Work out the finished part from the listing and answer in its coordinate system (mm). Face numbers are marked on the shaded views. A direction names the side the tool comes from. Coordinates: 2 decimals unless noted, no trailing zeros. Write each loop counter-clockwise with the first axis right and the second up, starting at its lowest first coordinate (ties: lowest second). Pieces come first, ordered by that corner, then holes. Notation, with made-up numbers: (-34, -16.5) - (18, -16.5) arc R28 ccw to (18, 4.5) - close; hole circle Ø9 at (-4.5, 16). An arc over 180 degrees is marked (long way). Use a Markdown table: item, result. Add a question column.
(1) The part is cut by section D-D, the plane x = 28. Give the vertices of the cut face in (y, z), then the cut area to 4 significant figures.
(2) The part is cut by section A-A, the plane x = 22. Give the vertices of the cut face in (y, z).
(3) For a pull along X with two mould halves and no side action, classify the marked faces 1, 2, 3 and 4 as released by +X, released by -X, zero draft, split by the parting line, or undercut.
(4) Find the intervals of material crossed by line 1 (Y direction, x = 13, z = 1.2); line 2 (Z direction, x = 17, y = 21); line 3 (X direction, y = 22.25, z = 3.9), in increasing order. Write a range as from..to.
(5) The part is cut by section C-C, the plane z = 4.35. Give the vertices of the cut face in (x, y), then the cut area to 3 significant figures.
(6) A tool of negligible diameter and unlimited length cuts with its end or side. For the marked faces 5 and 6, from which of +Z, -Z, +X, -X, +Y, -Y can it reach the whole face along a straight path? Write none if from no direction.
(7) Given pin 1 Ø1 at (x, y) = (27, 21.5) entering from -Z; pin 2 Ø0.7 at (y, z) = (18, 4) entering from +X; pin 3 Ø1.5 at (y, z) = (16.5, 1) entering from +X; pin 4 Ø1.9 at (y, z) = (18, 4) entering from -X, each flat-ended and moving along its own axis, determine where each tip first touches the part or whether it passes through.
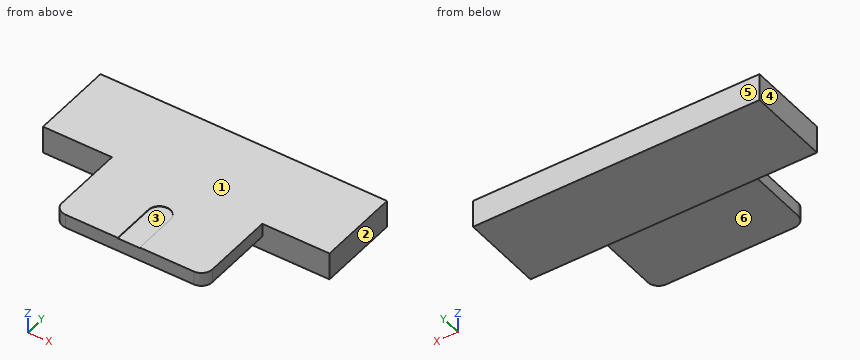
from build123d import *

# Parameters (mm, degrees)
BOX033_W          = 27.28
BOX033_H          = 15
BOX033_DEPTH      = 2.4
BOX031_W          = 10
BOX031_H          = 15
BOX031_DEPTH      = 5
BOX032_W          = 10
BOX032_H          = 15
BOX032_DEPTH      = 5
BOX030_W          = 4
BOX030_H          = 16
BOX030_DEPTH      = 10
CYLINDER023_R     = 2
CYLINDER023_DEPTH = 10
BOX029_W          = 8.2
BOX029_H          = 15
BOX029_DEPTH      = 10
BOX028_W          = 8.52
BOX028_H          = 15
BOX028_DEPTH      = 10
BOX027_W          = 44
BOX027_H          = 15
BOX027_DEPTH      = 2.6
BOX026_W          = 44
BOX026_H          = 30
BOX026_DEPTH      = 5
FILLET006_R       = 2


with BuildPart() as cube033:
    # Box033 → Box033 (new body)
    with BuildSketch(Plane(origin=(8.5, 21, 2.5), x_dir=(1, 0, 0), z_dir=(0, 0, 1))):
        with Locations((13.64, 7.5)):
            Rectangle(BOX033_W, BOX033_H)
    extrude(amount=BOX033_DEPTH)


with BuildPart() as cube031:
    # Box031 → Box031 (new body)
    with BuildSketch(Plane(origin=(-4, 36, 0), x_dir=(1, 0, 0), z_dir=(0, 0, 1))):
        with Locations((5, 7.5)):
            Rectangle(BOX031_W, BOX031_H)
    extrude(amount=BOX031_DEPTH)


with BuildPart() as cube032:
    # Box032 → Box032 (new body)
    with BuildSketch(Plane(origin=(38, 36, 0), x_dir=(1, 0, 0), z_dir=(0, 0, 1))):
        with Locations((5, 7.5)):
            Rectangle(BOX032_W, BOX032_H)
    extrude(amount=BOX032_DEPTH)


with BuildPart() as cube030:
    # Box030 → Box030 (new body)
    with BuildSketch(Plane(origin=(20, -8, 0), x_dir=(1, 0, 0), z_dir=(0, 0, 1))):
        with Locations((2, 8)):
            Rectangle(BOX030_W, BOX030_H)
    extrude(amount=BOX030_DEPTH)


with BuildPart() as fusion024:
    # Cylinder023 → Cylinder023 (new body)
    with BuildSketch(Plane(origin=(22, 8, 0), x_dir=(1, 0, 0), z_dir=(0, 0, 1))):
        Circle(CYLINDER023_R)
    extrude(amount=CYLINDER023_DEPTH)

    # Fusion024: union Cube030
    add(cube030.part)


with BuildPart() as cube029:
    # Box029 → Box029 (new body)
    with BuildSketch(Plane(origin=(35.8, 0, 0), x_dir=(1, 0, 0), z_dir=(0, 0, 1))):
        with Locations((4.1, 7.5)):
            Rectangle(BOX029_W, BOX029_H)
    extrude(amount=BOX029_DEPTH)


with BuildPart() as cube028:
    # Box028 → Box028 (new body)
    with BuildSketch(Plane.XY):
        with Locations((4.26, 7.5)):
            Rectangle(BOX028_W, BOX028_H)
    extrude(amount=BOX028_DEPTH)


with BuildPart() as cube027:
    # Box027 → Box027 (new body)
    with BuildSketch(Plane.XY):
        with Locations((22, 7.5)):
            Rectangle(BOX027_W, BOX027_H)
    extrude(amount=BOX027_DEPTH)


with BuildPart() as exterior_parte2_v2_base:
    # Box026 → Box026 (new body)
    with BuildSketch(Plane.XY):
        with Locations((22, 15)):
            Rectangle(BOX026_W, BOX026_H)
    extrude(amount=BOX026_DEPTH)

    # Cut007002012: cut Cube027
    add(cube027.part, mode=Mode.SUBTRACT)

    # Cut007002013: cut Cube028
    add(cube028.part, mode=Mode.SUBTRACT)

    # Cut007002014: cut Cube029
    add(cube029.part, mode=Mode.SUBTRACT)

    # Cut007002015: cut Fusion024
    add(fusion024.part, mode=Mode.SUBTRACT)


with BuildPart() as exterior_parte2_v2_base_1:
    # Cut007002015 placement: moved
    add(exterior_parte2_v2_base.part.moved(Location((0, 21, 0))))

    # Fusion025: union Cube031, Cube032
    add(cube031.part)
    add(cube032.part)

    # Fusion026: union Cube033
    add(cube033.part)

    # Fillet006
    fillet006_edges = [exterior_parte2_v2_base_1.edges().sort_by_distance(p)[0] for p in [
        (8.5, 21, 3.7),
        (35.8, 21, 3.8),
    ]]
    fillet(fillet006_edges, radius=FILLET006_R)


with BuildPart() as exterior_parte2_v2_base_2:
    # Fillet006 placement: moved
    add(exterior_parte2_v2_base_1.part.moved(Location((0, -12, 0.05))))


solid = exterior_parte2_v2_base_2.part
Model answer:
| question | item | result |
|---|---|---|
| 1 | outline | (9, 2.55) - (24, 2.55) - (24, 0.05) - (39, 0.05) - (39, 5.05) - (9, 5.05) - close |
| 1 | area | 112.5 mm^2 |
| 2 | outline | (9, 2.55) - (24, 2.55) - (24, 0.05) - (39, 0.05) - (39, 5.05) - (19, 5.05) - (19, 4.95) - (9, 4.95) - close |
| 3 | face 1 | zero draft |
| 3 | face 2 | released by +X |
| 3 | face 3 | undercut |
| 3 | face 4 | released by -X |
| 4 | line 1 | 24..39 |
| 4 | line 2 | 2.55..5.05 |
| 4 | line 3 | 8.5..35.8 |
| 5 | outline | (-4, 24) - (8.5, 24) - (8.5, 11) arc R2 ccw to (10.5, 9) - (33.8, 9) arc R2 ccw to (35.8, 11) - (35.8, 24) - (48, 24) - (48, 39) - (-4, 39) - close |
| 5 | area | 1,190 mm^2 |
| 6 | face 5 | +Z, -Z, +X, -X, +Y |
| 6 | face 6 | -Z, +X, -X, -Y |
| 7 | pin 1 | z = 2.55 |
| 7 | pin 2 | x = 35.8 |
| 7 | pin 3 | through |
| 7 | pin 4 | x = 8.5 |
